from build123d import *

# Parameters (mm, degrees)
SKETCH1_4_R         = 11
SKETCH1_4_R_2       = 2
SKETCH1_4_R_3       = 1.5
BOSS_EXTRUDE3_DEPTH = 4


with BuildPart() as part:
    # Sketch1_4 → Boss-Extrude3 (new body)
    with BuildSketch(Plane(origin=(0, 0, 0), x_dir=(1, 0, 0), z_dir=(0, 1, 0))):
        Polygon((130, -150), (170, -150), (170, 150), (130, 150), (130, 170), (-130, 170), (-130, 150), (-226, 150), (-226, -150), (-130, -150), (-130, -170), (130, -170), align=None)
        with Locations((135.829506597, -135.829506597)):
            Circle(SKETCH1_4_R, mode=Mode.SUBTRACT)
        with Locations((160, -95)):
            Circle(SKETCH1_4_R_2, mode=Mode.SUBTRACT)
        with Locations((160, 95)):
            Circle(SKETCH1_4_R_2, mode=Mode.SUBTRACT)
        with Locations((135.829506597, 135.829506597)):
            Circle(SKETCH1_4_R, mode=Mode.SUBTRACT)
        with Locations((85, -160)):
            Circle(SKETCH1_4_R_2, mode=Mode.SUBTRACT)
        with Locations((-85, -160)):
            Circle(SKETCH1_4_R_2, mode=Mode.SUBTRACT)
        with Locations((0, -160)):
            Circle(SKETCH1_4_R_2, mode=Mode.SUBTRACT)
        with Locations((85, 160)):
            Circle(SKETCH1_4_R_2, mode=Mode.SUBTRACT)
        with Locations((-85, 160)):
            Circle(SKETCH1_4_R_2, mode=Mode.SUBTRACT)
        with Locations((0, 160)):
            Circle(SKETCH1_4_R_2, mode=Mode.SUBTRACT)
        with BuildLine():
            Line((-161, 0), (-159, 0))
            ThreePointArc((-159, 0), (-157.585786438, -0.585786438), (-157, -2))
            Line((-157, -2), (-157, -68.911348687))
            ThreePointArc((-157, -68.911348687), (-157.585786438, -70.325562249), (-159, -70.911348687))
            Line((-159, -70.911348687), (-161, -70.911348687))
            ThreePointArc((-161, -70.911348687), (-162.414213562, -70.325562249), (-163, -68.911348687))
            Line((-163, -68.911348687), (-163, -2))
            ThreePointArc((-163, -2), (-162.414213562, -0.585786438), (-161, 0))
        make_face(mode=Mode.SUBTRACT)
        with Locations((-135.829506597, 135.829506597)):
            Circle(SKETCH1_4_R, mode=Mode.SUBTRACT)
        with Locations((-160, 95)):
            Circle(SKETCH1_4_R_2, mode=Mode.SUBTRACT)
        with Locations((-135.829506597, -135.829506597)):
            Circle(SKETCH1_4_R, mode=Mode.SUBTRACT)
        with Locations((-160, -95)):
            Circle(SKETCH1_4_R_2, mode=Mode.SUBTRACT)
        with Locations((-206.5, -139.5)):
            Circle(SKETCH1_4_R_3, mode=Mode.SUBTRACT)
        with Locations((-175.5, -139.5)):
            Circle(SKETCH1_4_R_3, mode=Mode.SUBTRACT)
        with Locations((-206.5, -108.5)):
            Circle(SKETCH1_4_R_3, mode=Mode.SUBTRACT)
        with Locations((-191, -124)):
            Circle(SKETCH1_4_R, mode=Mode.SUBTRACT)
        with Locations((-175.5, -108.5)):
            Circle(SKETCH1_4_R_3, mode=Mode.SUBTRACT)
        with Locations((-175.6, -51.5)):
            Circle(SKETCH1_4_R_2, mode=Mode.SUBTRACT)
        with Locations((-175.6, 98.5)):
            Circle(SKETCH1_4_R_2, mode=Mode.SUBTRACT)
    extrude(amount=BOSS_EXTRUDE3_DEPTH)


solid = part.part
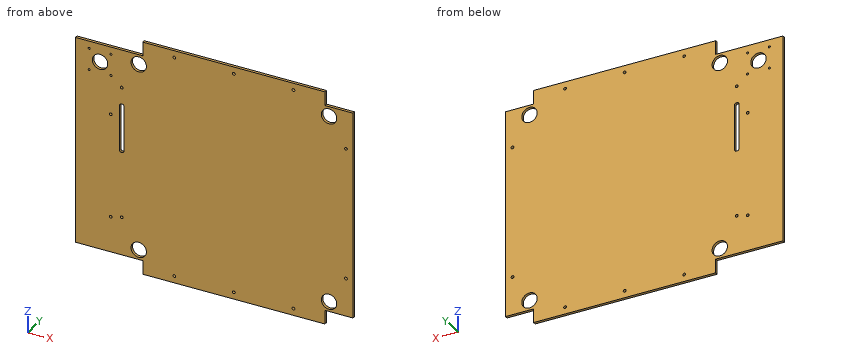
Source: CAD feature listing. Evaluate the final solid. Frame: model axes, mm. Give positions to 0.01 mm unless a question says otherwise; leave off trailing zeros. Write each loop counter-clockwise with the first axis right and the second up, starting at its lowest first coordinate (ties: lowest second). Pieces come first, ordered by that corner, then holes. Notation, with made-up numbers: M -2.5,73 L 48.5,73 A17 cw 48.5,96 Z; hole C 71,-14.5 d5. An arc over 180 degrees is marked long. Return JSON: item names as keys, results as strings. Group by question number.
1) Material intervals for line 1 along Z through (x, y) = (-206.5, 2.6); line 2 along Z through (x, y) = (85, 1.2); line 3 along X through (y, z) = (3.5, -94.5), sorted ascending. Write a range as [from, to].
2) Cut plane A-A, the plane x = -191. Output: boundary loops of the cut face in (y, z).
3) Cut plane B-B, the plane y = 1.75. Give the number of separate pieces and of enclosed holes in the cut face, plus the area to 3 significant figures.
4) Pin query (flat end, axial travel): P1, Ø5, axis at x = 85, z = -160, coming from the -Y side; P2, Ø1.8, axis at x = -206.5, z = 108.5, coming from the +Y side; P3, Ø2, axis at x = -171, y = 2, coming from the -Z side; P4, Ø2, axis at y = 2.5, z = 158, coming from the +X side. Return the tip coordinate at first contact, or that it passes through.
Recorded:
{
 "1": {"line 1": "z = [-150, 107], [110, 138], [141, 150]", "line 2": "z = [-170, -162], [-158, 158], [162, 170]", "line 3": "x = [-226, -161.94], [-158.06, 158.06], [161.94, 170]"},
 "2": {"outline": "M 0,-150 L 4,-150 L 4,113 L 0,113 Z; M 0,135 L 4,135 L 4,150 L 0,150 Z"},
 "3": {"separate pieces": "1", "enclosed holes": "22", "area": "127,000 mm²"},
 "4": {"P1": "stops at y = 0", "P2": "passes through", "P3": "stops at z = -150", "P4": "stops at x = 130"}
}
